Design review of the part built by this model. Coordinates are the model's own, in mm. Face numbers are marked on the shaded views. A direction names the side the tool comes from. Round coordinates to 2 decimals unless told otherwise and drop trailing zeros. Loops run counter-clockwise (first coordinate to the right, second up) from the corner with the lowest first, then second, coordinate; pieces in that order, holes last. Notation, with made-up numbers: M -34,-31.75 L -2,-31.75 A22 cw -2,-23.75 Z; hole C -37,-24 d10. An arc over 180 degrees is marked long. Use a Markdown table: item, result.
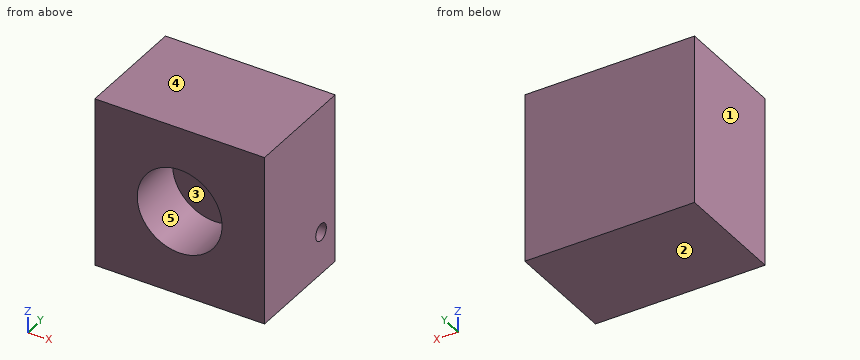
Autodesk Inventor part; units mm, degrees
ref_plane "YZ Plane" through (0, 0, 0) normal (1, 0, 0) x (0, 1, 0)
ref_plane "XZ Plane" through (0, 0, 0) normal (0, 1, 0) x (-1, 0, 0)
ref_plane "XY Plane" through (0, 0, 0) normal (0, 0, 1) x (1, 0, 0)
sketch "Sketch1" plane through (0, 0, 0) normal (0, 1, 0) x (-1, 0, 0)
  circle A0 centre (0, 0) radius 7.5
  line L0 (15, 15) -> (-15, 15)
  line L1 (-15, 15) -> (-15, -15)
  line L2 (-15, -15) -> (15, -15)
  line L3 (15, -15) -> (15, 15)
  dimension "d0" = 15
  dimension "d1" = 30
  dimension "d2" = 30
  dimension "d3" = 15
  dimension "d4" = 15
extrude "Extrusion1" add sketch "Sketch1" along normal blind 10
sketch "Sketch2" plane through (0, 10, 0) normal (0, 1, 0) x (1, 0, 0)
  line L0 (-15, -15) -> (15, -15)
  line L1 (15, -15) -> (15, 15)
  line L2 (15, 15) -> (-15, 15)
  line L3 (-15, 15) -> (-15, -15)
  point P0 (0, 0)
extrude "Extrusion2" add sketch "Sketch2" along normal blind 10
sketch "Sketch3" plane through (15, 0, 15) normal (1, 0, 0) x (0, 0, -1)
  line L0 (15, 0) -> (30, 0)
  line L1 (22.5, 10) -> (22.5, 0)
  line L2 (22.5, 0) -> (22.5, 7)
  circle A0 centre (22.5, 16) radius 1.5
  dimension "d9" = 16
  dimension "d10" = 3
extrude "Extrusion3" cut sketch "Sketch3" against normal blind 5
properties part number "bruh2"
1. The part is to be moulded in two halves that separate along X. For the marked faces 1, 2 and 3, say which applies: pulls with the +X half, pulls with the -X half, needs draft (parallel to the pull), parting line crosses it, or undercut.
Check values:
| item | result |
|---|---|
| face 1 | pulls with the -X half |
| face 2 | needs draft |
| face 3 | undercut |
2. Take a section at C-C on y = 8.25. Give the boundary of the cut face in (x, z), and give its area (3 significant figures).
Check values:
| item | result |
|---|---|
| outline | M -15,-15 L 15,-15 L 15,15 L -15,15 Z; hole C 0,0 d15 |
| area | 723 mm² |
3. Insertion check: pin 1 (4.5 mm diameter, centred on x = -0.5, z = -2.5, fed in from -Y). The pin has a flat end and moves straight along its axis. Give the tip position at first contact, or say it passes through.
Check values:
| item | result |
|---|---|
| pin 1 | stops at y = 10 |
4. Take a section at A-A on y = 16. Give the boundary of the cut face in (x, z), and give its area (3 significant figures).
Check values:
| item | result |
|---|---|
| outline | M -15,-15 L 15,-15 L 15,-9 L 10,-9 L 10,-6 L 15,-6 L 15,15 L -15,15 Z |
| area | 885 mm² |
5. Take a section at B-B on z = 0. Give the boundary of the cut face in (x, y).
Check values:
| item | result |
|---|---|
| outline | M -15,0 L -7.5,0 L -7.5,10 L 7.5,10 L 7.5,0 L 15,0 L 15,20 L -15,20 Z |
6. Machinability: for the marked faces 4 and 5, which of the approach directions +Z, -Z, +X, -X, +Y, -Y give a long, thin tool a straight path to every point of the face, cutting with its end or side? Answer none if there is none.
Check values:
| item | result |
|---|---|
| face 4 | +Z, +X, -X, +Y, -Y |
| face 5 | -Y |
7. Wall thickness on line 1 along Z through (x, y) = (0, 8.25); line 2 along Y through (x, z) = (12.9, -7.5); line 3 along Y through (x, z) = (4.5, -3.25): over which ranges is each line inside the solid? List them lowest first. Write a range as from..to.
Check values:
| item | result |
|---|---|
| line 1 | z = -15..-7.5, 7.5..15 |
| line 2 | y = 0..14.5, 17.5..20 |
| line 3 | y = 10..20 |
